```python
from build123d import *

# Parameters (mm, degrees)
SKETCH1_R           = 12.475
BOSS_EXTRUDE1_DEPTH = 10.5
SKETCH6_R           = 12.475
BOSS_EXTRUDE7_DEPTH = 4.5
SKETCH3_R           = 17
BOSS_EXTRUDE3_DEPTH = 1
SKETCH4_R           = 7.5
BOSS_EXTRUDE5_DEPTH = 0.5
SKETCH5_R           = 3.9625
BOSS_EXTRUDE6_DEPTH = 7
BOSS_EXTRUDE8_START = 5.5
BOSS_EXTRUDE8_DEPTH = 5.5
CHAMFER1_SIZE       = 0.5
FILLET1_R           = 0.25


with BuildPart() as part:
    # Sketch1 → Boss-Extrude1 (new body)
    # profile 1 of 2: a face of its own
    with BuildSketch(Plane.XY):
        with BuildLine():
            Line((-4, 0), (-2, 3.464101615))
            ThreePointArc((-2, 3.464101615), (-3.464101615, 2), (-4, 0))
        make_face()
    # profile 2 of 2: a face of its own
    with BuildSketch(Plane.XY):
        with Locations(Location((-2.17, 0, 0), (0, 0, 180))):
            Circle(SKETCH1_R)
        Polygon((1.985566243, -3.439101615), (3.971132487, 0), (1.985566243, 3.439101615), (-1.985566243, 3.439101615), (-3.971132487, 0), (-1.985566243, -3.439101615), align=None, mode=Mode.SUBTRACT)
    extrude(amount=BOSS_EXTRUDE1_DEPTH)

    # Sketch6 → Boss-Extrude7 (add)
    with BuildSketch(Plane.XY.offset(10.5)):
        with Locations(Location((-2.17, 0, 0), (0, 0, 180))):
            Circle(SKETCH6_R)
    extrude(amount=BOSS_EXTRUDE7_DEPTH)

    # Sketch3 → Boss-Extrude3 (add)
    with BuildSketch(Plane(origin=(0, 0, 15), x_dir=(-1, 0, 0), z_dir=(0, 0, -1))):
        with Locations((2.17, 0)):
            Circle(SKETCH3_R)
    extrude(amount=-BOSS_EXTRUDE3_DEPTH)

    # Sketch4 → Boss-Extrude5 (add)
    with BuildSketch(Plane.XY.offset(16)):
        Circle(SKETCH4_R)
    extrude(amount=BOSS_EXTRUDE5_DEPTH)

    # Sketch5 → Boss-Extrude6 (add)
    with BuildSketch(Plane.XY.offset(16.5)):
        Circle(SKETCH5_R)
    extrude(amount=BOSS_EXTRUDE6_DEPTH)

    # Sketch7 → Boss-Extrude8 (add)
    with BuildSketch(Plane(origin=(0, 0, 0), x_dir=(-1, 0, 0), z_dir=(0, 0, -1)).offset(BOSS_EXTRUDE8_START)):
        with BuildLine():
            ThreePointArc((14.645, 0), (10.206747632, 9.541295116), (0.05, 12.293544037))
            Line((0.05, 12.293544037), (0.05, 3.439101615))
            Line((0.05, 3.439101615), (1.985566243, 3.439101615))
            Line((1.985566243, 3.439101615), (3.971132487, 0))
            Line((3.971132487, 0), (1.985566243, -3.439101615))
            Line((1.985566243, -3.439101615), (0.05, -3.439101615))
            Line((0.05, -3.439101615), (0.05, -12.293544037))
            ThreePointArc((0.05, -12.293544037), (10.206747632, -9.541295116), (14.645, 0))
        make_face()
    extrude(amount=-BOSS_EXTRUDE8_DEPTH)

    # Chamfer1
    chamfer1_edges = [part.edges().sort_by_distance(p)[0] for p in [
        (-3.9625, 0, 23.5),
    ]]
    chamfer(chamfer1_edges, length=CHAMFER1_SIZE)

    # Fillet1
    fillet1_edges = [part.edges().sort_by_distance(p)[0] for p in [
        (-0.05, 7.866322826, -5.5),
        (-0.05, -7.866322826, -5.5),
    ]]
    fillet(fillet1_edges, radius=FILLET1_R)


solid = part.part
```
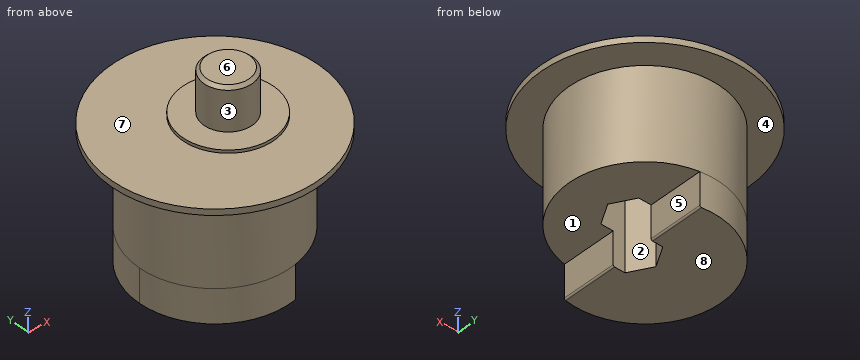
Geometry: final body of the model. Coordinates: model frame, mm. Face numbers are marked on the shaded views. A direction names the side the tool comes from. Coordinates: 2 decimals unless noted, no trailing zeros. Order: outer loops, then holes, each group sorted by start corner. A loop starts at its lowest first (then second) coordinate and runs counter-clockwise, first axis right, second up.
Item 1: Material intervals for line 1 along Y through (x, z) = (1, 3); line 2 along Z through (x, y) = (-13, 11); line 3 along Z through (x, y) = (-9, -2), sorted ascending.
Answer:
line 1: y = -12.07 to -3.44, 3.44 to 12.07
line 2: z = 15 to 16
line 3: z = -5.5 to 16
Item 2: Section query C-C (y = -11.5). Output: boundary loops of the cut face in (x, z).
Answer:
outline: (-14.69, 15) - (-7, 15) - (-7, -5.5) - (-0.3, -5.5) arc R0.25 ccw to (-0.05, -5.25) - (-0.05, 0) - (2.66, 0) - (2.66, 15) - (10.35, 15) - (10.35, 16) - (-14.69, 16) - close
Item 3: Draft query along Y for the marked faces 1, 2 and 3. Return one class per face: released by +Y, released by -Y, zero draft, split by the parting line, or undercut.
Answer:
face 1: zero draft
face 2: undercut
face 3: split by the parting line
Item 4: Section query B-B (x = -8.5). Output: boundary loops of the cut face in (y, z).
Answer:
outline: (-15.78, 15) - (-10.75, 15) - (-10.75, -5.5) - (10.75, -5.5) - (10.75, 15) - (15.78, 15) - (15.78, 16) - (-15.78, 16) - close
Item 5: Section query A-A (z = 3). Output: boundary loops of the cut face in (x, y) (3 decimals), then the cut area to 3 significant figures.
Answer:
outline: circle Ø24.95 at (-2.17, 0); hole (-3.971, 0) - (-1.986, -3.439) - (1.986, -3.439) - (3.971, 0) - (1.986, 3.439) - (-1.986, 3.439) - close
area: 448 mm2
Item 6: Contact query for flat-ended pins moving along their axis: P1, Ø1.5, axis at x = 5, z = 13.5, coming from the +Y side; P2, Ø6, axis at x = -6, z = 13.5, coming from the +Y side; P3, Ø10, axis at x = 10, z = -0.5, coming from the -Y side. Output: stop coordinate, or through.
Answer:
P1: stops at y = 10.7
P2: stops at y = 16.96
P3: stops at y = -10.19
Item 7: Access query for the marked faces 4, 5, 6, 7 and 8. Directions: +Z, -Z, +X, -X, +Y, -Y. A direction counts if a zero-diameter tool reaches every point of the face in a straight line with its end or side. Return the directions, or none.
Answer:
face 4: -Z
face 5: -Z, +X, +Y, -Y
face 6: +Z, +X, -X, +Y, -Y
face 7: +Z
face 8: -Z, +X, -X, +Y, -Y
Item 8: Section query D-D (z = 17). Output: boundary loops of the cut face in (x, y) (1 decimal), then the cut area to 3 significant figures.
Answer:
outline: circle Ø7.9 at (0, 0)
area: 49.3 mm2
